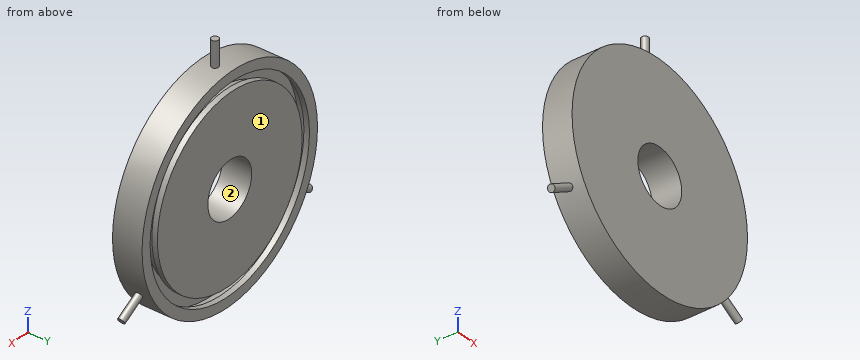
```python
from build123d import *

# Parameters (mm, degrees)
SKETCH1_R           = 30
SKETCH1_R_2         = 7.5
BOSS_EXTRUDE1_DEPTH = 4
BOSS_EXTRUDE2_START = 29
SKETCH3_R           = 0.95
BOSS_EXTRUDE2_DEPTH = 8
CIRPATTERN1_COUNT   = 3


with BuildPart() as part:
    # Sketch1 → Boss-Extrude1 (new, symmetric)
    with BuildSketch(Plane(origin=(0, 0, 0), x_dir=(1, 0, 0), z_dir=(0, 1, 0))):
        with Locations(Location((0, 0, 0), (0, 0, 270))):
            Circle(SKETCH1_R)
        with Locations(Location((0, 0, 0), (0, 0, 270))):
            Circle(SKETCH1_R_2, mode=Mode.SUBTRACT)
    extrude(amount=BOSS_EXTRUDE1_DEPTH, both=True)

    # Sketch2 → Cut-Revolve2 (revolve, cut)
    with BuildSketch(Plane(origin=(0, 0, 0), x_dir=(0, 0, -1), z_dir=(1, 0, 0))):
        Polygon((-27.25, 4), (-24.75, 4), (-24.75, 2.5), (-23.5, 2.5), (-23.5, -0.04), (-28.5, -0.04), (-28.5, 2.5), (-27.25, 2.5), align=None)
    revolve(axis=Axis((0, 8.260026976, 0), (0, -1, 0)), mode=Mode.SUBTRACT)

    # Sketch3 → Boss-Extrude2 (add)
    with BuildSketch(Plane.XY.offset(BOSS_EXTRUDE2_START)):
        with Locations(Location((0, 0, 0), (0, 0, 180))):
            Circle(SKETCH3_R)
    boss_extrude2 = extrude(amount=BOSS_EXTRUDE2_DEPTH)

    # CirPattern1: Boss-Extrude2 ×3 about axis
    cirpattern1_axis = Axis((0, 0, 0), (0, 1, 0))
    for i in range(1, CIRPATTERN1_COUNT):
        add(boss_extrude2.rotate(cirpattern1_axis, i * 360 / CIRPATTERN1_COUNT))


solid = part.part
```
Check sheet for the modelled part. Datum: model origin and axes. Units: mm. Face numbers are marked on the shaded views. Give positions to 0.01 mm unless a question says otherwise; leave off trailing zeros. Write each loop counter-clockwise with the first axis right and the second up, starting at its lowest first coordinate (ties: lowest second). Pieces come first, ordered by that corner, then holes. Notation, with made-up numbers: (69, 22.25) -> (126, 22.25) arc R13 ccw to (126, 26.25) -> close; hole circle Ø1 at (27, 62). An arc over 180 degrees is marked (long way). Use CSV: the item, a comma, the result in double quotes. Start each with the question number.
Q1. Cross-section at B-B on z = 0. Enter the section's corners in (x, y), and give its area (3 significant figures).
Q2. Scan lines: line 1 along Z through (x, y) = (-1, 3.75); line 2 along Y through (x, z) = (5, -27); line 3 along X through (y, z) = (3.5, 13.5). Record each from-to range of solid material in increasing order.
Q3. Cross-section at D-D on y = -2. Enter the section's corners in (x, z).
Q4. Release check for a two-part mould opening along Z. For the marked faces 1 and 2 record: +Z half, -Z half, draft (parallel to the pull), parting line (faces both ways), or undercut.
Q5. Cross-section at A-A on x = 0. Enter the section's corners in (y, z).
Q6. Cross-section at C-C on x = 10.5. Enter the section's corners in (y, z).
Q7. Depth check by flat-ended pin: P1, Ø2, axis at y = 2.5, z = -3.5, coming from the -X side; P2, Ø2, axis at x = -6.5, y = 2, coming from the -Z side; P3, Ø4, axis at y = 0, z = 6, coming from the +X side. Enter the tip coordinate at first touch or a pass-through.
Working result:
1,outline,"(-30, -4) -> (-7.5, -4) -> (-7.5, 4) -> (-24.75, 4) -> (-24.75, 2.5) -> (-23.5, 2.5) -> (-23.5, -0.04) -> (-28.5, -0.04) -> (-28.5, 2.5) -> (-27.25, 2.5) -> (-27.25, 4) -> (-30, 4) -> close; (7.5, -4) -> (30, -4) -> (30, 4) -> (27.25, 4) -> (27.25, 2.5) -> (28.5, 2.5) -> (28.5, -0.04) -> (23.5, -0.04) -> (23.5, 2.5) -> (24.75, 2.5) -> (24.75, 4) -> (7.5, 4) -> close"
1,area,"327 mm^2"
2,line 1,"z = -29.98 to -27.23, -24.73 to -7.43, 7.43 to 24.73, 27.23 to 29.98"
2,line 2,"y = -4 to -0.04, 2.5 to 4"
2,line 3,"x = -26.79 to -23.67, -20.74 to 20.74, 23.67 to 26.79"
3,outline,"circle Ø60 at (0, 0); hole circle Ø15 at (0, 0)"
4,face 1,"draft"
4,face 2,"undercut"
5,outline,"(-4, -30) -> (4, -30) -> (4, -27.25) -> (2.5, -27.25) -> (2.5, -28.5) -> (-0.04, -28.5) -> (-0.04, -23.5) -> (2.5, -23.5) -> (2.5, -24.75) -> (4, -24.75) -> (4, -7.5) -> (-4, -7.5) -> close; (-4, 7.5) -> (4, 7.5) -> (4, 24.75) -> (2.5, 24.75) -> (2.5, 23.5) -> (-0.04, 23.5) -> (-0.04, 28.5) -> (2.5, 28.5) -> (2.5, 27.25) -> (4, 27.25) -> (4, 30) -> (0.95, 30) -> (0.95, 37) -> (-0.95, 37) -> (-0.95, 30) -> (-4, 30) -> close"
6,outline,"(-4, -28.1) -> (4, -28.1) -> (4, -25.15) -> (2.5, -25.15) -> (2.5, -26.5) -> (-0.04, -26.5) -> (-0.04, -21.02) -> (2.5, -21.02) -> (2.5, -22.41) -> (4, -22.41) -> (4, 22.41) -> (2.5, 22.41) -> (2.5, 21.02) -> (-0.04, 21.02) -> (-0.04, 26.5) -> (2.5, 26.5) -> (2.5, 25.15) -> (4, 25.15) -> (4, 28.1) -> (-4, 28.1) -> close"
7,P1,"stops at x = -29.9"
7,P2,"stops at z = -29.49"
7,P3,"stops at x = 29.73"
